```python
from build123d import *

# Parameters (mm, degrees)
SKETCH2_W               = 76.2
SKETCH2_H               = 25.4
BOSS_EXTRUDE1_DEPTH     = 25.4
SKETCH3_W               = 38.1
SKETCH3_H               = 6.35
CUT_EXTRUDE1_DEPTH      = 65.757547823
CUT_EXTRUDE2_DEPTH      = 48.519048812
CUT_EXTRUDE2_DEPTH_BACK = 48.519048812
SKETCH4_W               = 31.75
SKETCH4_H               = 31.75
FILLET2_R               = 15.875
SKETCH5_R               = 15.875
BOSS_EXTRUDE2_DEPTH     = 6.35
HOLE1_D                 = 9.525
HOLE1_DEPTH             = 31.75
HOLE1_CBORE_D           = 19.05
HOLE1_CBORE_DEPTH       = 6.35
HOLE1_TIP               = 2.861598698


with BuildPart() as part:
    # Sketch2 → Boss-Extrude1 (new, symmetric)
    with BuildSketch(Plane.XY):
        Rectangle(SKETCH2_W, SKETCH2_H)
    extrude(amount=BOSS_EXTRUDE1_DEPTH, both=True)

    # Sketch3 → Cut-Extrude1 (cut, through all)
    with BuildSketch(Plane.XY.offset(25.4)):
        with Locations((19.05, -9.525)):
            Rectangle(SKETCH3_W, SKETCH3_H)
    extrude(amount=-CUT_EXTRUDE1_DEPTH, mode=Mode.SUBTRACT)

    # Sketch4 → Cut-Extrude2 (cut, two sides: drawn at the far end of the back side and taken through both)
    with BuildSketch(Plane(origin=(0, 0, 0), x_dir=(1, 0, 0), z_dir=(0, 1, 0)).offset(-CUT_EXTRUDE2_DEPTH_BACK)):
        with Locations((22.225, 0)):
            Rectangle(SKETCH4_W, SKETCH4_H)
    extrude(amount=CUT_EXTRUDE2_DEPTH + CUT_EXTRUDE2_DEPTH_BACK, mode=Mode.SUBTRACT)

    # Fillet2
    fillet2_edges = [part.edges().sort_by_distance(p)[0] for p in [
        (6.35, 3.175, 15.875),
        (6.35, 3.175, -15.875),
    ]]
    fillet(fillet2_edges, radius=FILLET2_R - 0.0001)  # a hair under: the kernel refuses the full size

    # Sketch5 → Boss-Extrude2 (add)
    with BuildSketch(Plane(origin=(0, 12.7, 0), x_dir=(1, 0, 0), z_dir=(0, 1, 0))):
        with Locations(Location((-19.05, 0, 0), (0, 0, 90))):
            Circle(SKETCH5_R)
    extrude(amount=BOSS_EXTRUDE2_DEPTH)

    # Hole1
    with Locations(Plane(origin=(-19.05, 19.05, 0), x_dir=(0, 0, 1), z_dir=(0, 1, 0))):
        with Locations((0, 0)):
            CounterBoreHole(HOLE1_D / 2, HOLE1_CBORE_D / 2, HOLE1_CBORE_DEPTH, depth=HOLE1_DEPTH)
            with Locations((0, 0, -(HOLE1_DEPTH + HOLE1_TIP / 2))):  # 118° drill point
                Cone(0, HOLE1_D / 2, HOLE1_TIP, mode=Mode.SUBTRACT)


solid = part.part
```
Verification items for the finished model (mm, model axes). A direction names the side the tool comes from. Coordinates: 2 decimals unless noted, no trailing zeros. Order: outer loops, then holes, each group sorted by start corner. A loop starts at its lowest first (then second) coordinate and runs counter-clockwise, first axis right, second up. Notation, with made-up numbers: (5, 62) - (45, 62) arc R24 cw to (45, 98) - close; hole circle Ø10 at (13.25, -22). An arc over 180 degrees is marked (long way). Return JSON: item names as keys, results as strings.
(1) Section check D-D, the plane x = -4. Record the cut outline in (y, z), and give its area (3 significant figures).
Filled sheet:
{"outline": "(-12.7, -25.4) - (12.7, -25.4) - (12.7, -5.05) - (19.05, -5.05) - (19.05, 5.05) - (12.7, 5.05) - (12.7, 25.4) - (-12.7, 25.4) - close", "area": "1,350 mm^2"}
(2) Mould release check, pull along X, two halves, no side actions. Record for faces 1 (the flat face through (0, -10, 0)), 2 (the cylindrical face through (-14.33, -0.18, 0.62)), 3 (the flat face through (30, 3, -15.875)): pulls with the +X half, pulls with the -X half, needs draft (parallel to the pull), parting line crosses it, or undercut.
Filled sheet:
{"face 1": "pulls with the +X half", "face 2": "undercut", "face 3": "needs draft"}
(3) Section check C-C, the plane z = 7. Record the cut outline in (x, y).
Filled sheet:
{"outline": "(-38.1, -12.7) - (0, -12.7) - (0, -6.35) - (7.98, -6.35) - (7.98, 12.7) - (-4.8, 12.7) - (-4.8, 19.05) - (-12.59, 19.05) - (-12.59, 12.7) - (-25.51, 12.7) - (-25.51, 19.05) - (-33.3, 19.05) - (-33.3, 12.7) - (-38.1, 12.7) - close"}
(4) Access from +Z, -Z, +X, -X, +Y, -Y to the whole of each face (thin tool, end or side, straight path). Record for faces 4 (the flat face through (-38.1, 0, 0)), 5 (the flat face through (6, -6.35, 0)), 6 (the cylindrical face through (-3.553, 15.831, 3.441)), 7 (the cylindrical face through (11.124, 3.308, 11.348)), 8 (the flat face through (-19, -12.7, 6)).
Filled sheet:
{"face 4": "+Z, -Z, -X, +Y, -Y", "face 5": "+Z, -Z, +X, -Y", "face 6": "+Y", "face 7": "+X, +Y, -Y", "face 8": "+Z, -Z, +X, -X, -Y"}
(5) Section check A-A, the plane x = 33.5. Record the cut outline in (y, z) (3 decimals).
Filled sheet:
{"outline": "(-6.35, -25.4) - (12.7, -25.4) - (12.7, -15.875) - (-6.35, -15.875) - close; (-6.35, 15.875) - (12.7, 15.875) - (12.7, 25.4) - (-6.35, 25.4) - close"}
(6) Go/stop test with flat-tipped pins: pin 1 (1 mm diameter, centred on x = 30, z = 14, fed in from -Y); pin 2 (10 mm diameter, centred on x = 14, z = -9, fed in from +Y); pin 3 (1 mm diameter, centred on x = 28, z = -16, fed in from -Y); pin 4 (5 mm diameter, centred on y = -9, z = -6, fed in from +X). Record where each tip stops, or that it passes through.
Filled sheet:
{"pin 1": "passes through", "pin 2": "stops at y = 12.7", "pin 3": "stops at y = -6.35", "pin 4": "stops at x = 0"}
(7) Thickness scan on line 1 along Z through (x, y) = (24, 9.5) (3 decimals); line 2 along X through (y, z) = (16.25, 0) (3 decimals); line 3 along X through (y, z) = (4.75, 0). Record the ranges inside material, lowest first.
Filled sheet:
{"line 1": "z = -25.4 to -15.875, 15.875 to 25.4", "line 2": "x = -34.925 to -28.575, -9.525 to -3.175", "line 3": "x = -38.1 to -23.81, -14.29 to 6.35"}
